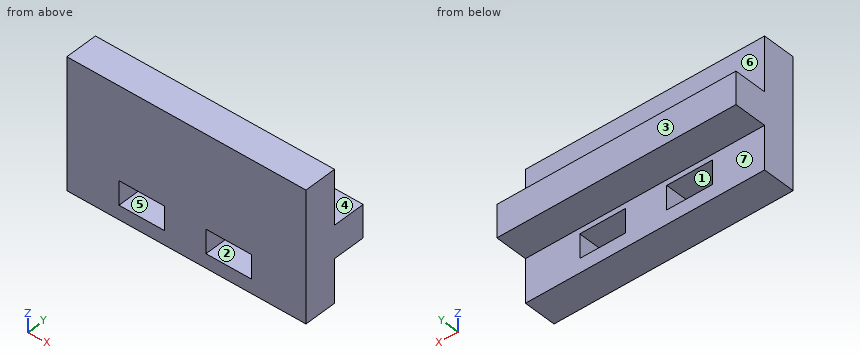
```python
from build123d import *

# Parameters (mm, degrees)
SKETCH_232_W          = 210
SKETCH_232_H          = 53
EXTRUDE_1_DEPTH       = 50
SKETCH_3_W            = 200
SKETCH_3_H            = 43
CUT_EXTRUDE_1_DEPTH   = 45
SKETCH_4_R            = 3.5
EXTRUDE_2_DEPTH       = 2
EXTRUDE_2_TAPER       = 1
FILLET_2_R            = 0.5
SKETCH_4_5_R          = 3.5
EXTRUDE_3_DEPTH       = 2
SKETCH_4_6_R          = 3.5
EXTRUDE_4_DEPTH       = 2
SKETCH_4_7_R          = 3.5
EXTRUDE_5_DEPTH       = 2
FILLET_3_R            = 0.5
FILLET_4_R            = 0.5
FILLET_5_R            = 0.5
SKETCH_7_R            = 6
CUT_EXTRUDE_2_DEPTH   = 14
CUT_EXTRUDE_2_DRAFT   = -5
FILLET_6_R            = 2
SKETCH_8_R            = 7
EXTRUDE_6_DEPTH       = 7
EXTRUDE_6_TAPER       = 5
SKETCH_9_R            = 5.15
CUT_EXTRUDE_3_DEPTH   = 7
CUT_EXTRUDE_3_DRAFT   = 5
SKETCH_10_W           = 29.4
SKETCH_10_H           = 26.3
CUT_EXTRUDE_4_DEPTH   = 5
SKETCH_13_W           = 39.2
SKETCH_13_H           = 27.5
CUT_EXTRUDE_5_DEPTH   = 2
SKETCH_14_W           = 6
SKETCH_14_H           = 6
CUT_EXTRUDE_6_DEPTH   = 5
FILLET_7_R            = 2
EXTRUDE_8_DEPTH       = 3
SKETCH_18_W           = 200
SKETCH_18_H           = 43
SKETCH_18_W_2         = 194
SKETCH_18_H_2         = 37
EXTRUDE_4672_DEPTH    = 3
SKETCH_21_W           = 4.2
SKETCH_21_H           = 2.2
CUT_EXTRUDE_7_DEPTH   = 3
SKETCH_23_OUTSIDE_W   = 255.334
SKETCH_23_OUTSIDE_H   = 98.334
SKETCH_23_OUTSIDE_W_2 = 22
SKETCH_23_OUTSIDE_H_2 = 12
CUT_EXTRUDE_8_DEPTH   = 6


with BuildPart() as part:
    # Sketch 232 → Бобышка-Вытянуть1 (new body)
    with BuildSketch(Plane(origin=(0, 0, 0), x_dir=(1, 0, 0), z_dir=(0, 1, 0))):
        Rectangle(SKETCH_232_W, SKETCH_232_H)
    extrude(amount=EXTRUDE_1_DEPTH)

    # Эскиз3 → Вырез-Вытянуть1 (cut)
    with BuildSketch(Plane.XZ):
        Rectangle(SKETCH_3_W, SKETCH_3_H)
    extrude(amount=-CUT_EXTRUDE_1_DEPTH, mode=Mode.SUBTRACT)

    # Эскиз4 → Бобышка-Вытянуть2 (add)
    with BuildSketch(Plane(origin=(0, 50, 0), x_dir=(1, 0, 0), z_dir=(0, 1, 0))):
        with Locations((98, 19.5)):
            Circle(SKETCH_4_R)
    extrude(amount=EXTRUDE_2_DEPTH, taper=EXTRUDE_2_TAPER)

    # Скругление2
    fillet_2_edges = [part.edges().sort_by_distance(p)[0] for p in [
        (94.53491013, 52, -19.5),
    ]]
    fillet(fillet_2_edges, radius=FILLET_2_R)

    # Эскиз4<5> → Бобышка-Вытянуть3 (add)
    with BuildSketch(Plane(origin=(0, 50, 0), x_dir=(1, 0, 0), z_dir=(0, 1, 0))):
        with Locations(Location((98, -19.5, 0), (0, 0, 90))):
            Circle(SKETCH_4_5_R)
    extrude(amount=EXTRUDE_3_DEPTH)

    # Эскиз4<6> → Бобышка-Вытянуть4 (add)
    with BuildSketch(Plane(origin=(0, 50, 0), x_dir=(1, 0, 0), z_dir=(0, 1, 0))):
        with Locations(Location((-98, -19.5, 0), (0, 0, 270))):
            Circle(SKETCH_4_6_R)
    extrude(amount=EXTRUDE_4_DEPTH)

    # Эскиз4<7> → Бобышка-Вытянуть5 (add)
    with BuildSketch(Plane(origin=(0, 50, 0), x_dir=(1, 0, 0), z_dir=(0, 1, 0))):
        with Locations(Location((-98, 19.5, 0), (0, 0, 90))):
            Circle(SKETCH_4_7_R)
    extrude(amount=EXTRUDE_5_DEPTH)

    # Скругление3
    fillet_3_edges = [part.edges().sort_by_distance(p)[0] for p in [
        (-98, 52, 16),
    ]]
    fillet(fillet_3_edges, radius=FILLET_3_R)

    # Скругление4
    fillet_4_edges = [part.edges().sort_by_distance(p)[0] for p in [
        (-98, 52, -16),
    ]]
    fillet(fillet_4_edges, radius=FILLET_4_R)

    # Скругление5
    fillet_5_edges = [part.edges().sort_by_distance(p)[0] for p in [
        (98, 52, 23),
    ]]
    fillet(fillet_5_edges, radius=FILLET_5_R)


with BuildPart() as cut_extrude_2_tool:
    # Эскиз7 → Вырез-Вытянуть2 (with draft: the straight prism first)
    with BuildSketch(Plane(origin=(0, 0, -26.5), x_dir=(-1, 0, 0), z_dir=(0, 0, -1))):
        with Locations((0, 35.081888724)):
            Circle(SKETCH_7_R)
    extrude(amount=-CUT_EXTRUDE_2_DEPTH)
    # Вырез-Вытянуть2: the draft: its side faces are tilted about the plane it starts from
    cut_extrude_2_sides = [cut_extrude_2_tool.faces().sort_by_distance(p)[0] for p in [
        (6, 35.081888724, -19.5),
    ]]
    draft(cut_extrude_2_sides, Plane(origin=(0, 0, -26.5), x_dir=(-1, 0, 0), z_dir=(0, 0, -1)), CUT_EXTRUDE_2_DRAFT)


with BuildPart() as part_1:
    add(part.part)

    # Вырез-Вытянуть2: cut by cut_extrude_2_tool
    add(cut_extrude_2_tool.part, mode=Mode.SUBTRACT)

    # Скругление6
    fillet_6_edges = [part_1.edges().sort_by_distance(p)[0] for p in [
        (6, 35.081888724, -26.5),
    ]]
    fillet(fillet_6_edges, radius=FILLET_6_R)

    # Эскиз8 → Бобышка-Вытянуть6 (add)
    with BuildSketch(Plane.XY.offset(-21.5)):
        with Locations((0, 35.081888724)):
            Circle(SKETCH_8_R)
    extrude(amount=EXTRUDE_6_DEPTH, taper=EXTRUDE_6_TAPER)


with BuildPart() as cut_extrude_3_tool:
    # Эскиз9 → Вырез-Вытянуть3 (with draft: the straight prism first)
    with BuildSketch(Plane.XY.offset(-14.5)):
        with Locations((0, 35.081888724)):
            Circle(SKETCH_9_R)
    extrude(amount=-CUT_EXTRUDE_3_DEPTH)
    # Вырез-Вытянуть3: the draft: its side faces are tilted about the plane it starts from
    cut_extrude_3_sides = [cut_extrude_3_tool.faces().sort_by_distance(p)[0] for p in [
        (-5.15, 35.081888724, -18),
    ]]
    draft(cut_extrude_3_sides, Plane.XY.offset(-14.5), CUT_EXTRUDE_3_DRAFT)


with BuildPart() as part_2:
    add(part_1.part)

    # Вырез-Вытянуть3: cut by cut_extrude_3_tool
    add(cut_extrude_3_tool.part, mode=Mode.SUBTRACT)

    # Эскиз10 → Вырез-Вытянуть4 (cut)
    with BuildSketch(Plane.XY.offset(26.5)):
        with Locations((-50, 25)):
            Rectangle(SKETCH_10_W, SKETCH_10_H)
    extrude(amount=-CUT_EXTRUDE_4_DEPTH, mode=Mode.SUBTRACT)

    # Эскиз13 → Вырез-Вытянуть5 (cut)
    with BuildSketch(Plane(origin=(0, 0, 21.5), x_dir=(-1, 0, 0), z_dir=(0, 0, -1))):
        with Locations((50, 25)):
            Rectangle(SKETCH_13_W, SKETCH_13_H)
    extrude(amount=-CUT_EXTRUDE_5_DEPTH, mode=Mode.SUBTRACT)

    # Эскиз14 → Вырез-Вытянуть6 (cut)
    with BuildSketch(Plane.XY.offset(26.5)):
        with Locations((-76.5, 31.8)):
            Rectangle(SKETCH_14_W, SKETCH_14_H)
        with Locations((-76.5, 18.2)):
            Rectangle(SKETCH_14_W, SKETCH_14_H)
    extrude(amount=-CUT_EXTRUDE_6_DEPTH, mode=Mode.SUBTRACT)

    # Скругление7
    fillet_7_edges = [part_2.edges().sort_by_distance(p)[0] for p in [
        (-105, 50, 0),
        (0, 50, 26.5),
        (105, 50, 0),
        (105, 25, 26.5),
        (-105, 25, 26.5),
        (-105, 25, -26.5),
        (105, 25, -26.5),
        (0, 50, -26.5),
    ]]
    fillet(fillet_7_edges, radius=FILLET_7_R)


with BuildPart() as body_2:
    # Эскиз17 → Бобышка-Вытянуть8 (new body)
    with BuildSketch(Plane.XZ):
        with BuildLine():
            Line((-105, 24.5), (-105, -24.5))
            ThreePointArc((-105, -24.5), (-104.414213562, -25.914213562), (-103, -26.5))
            Line((-103, -26.5), (103, -26.5))
            ThreePointArc((103, -26.5), (104.414213562, -25.914213562), (105, -24.5))
            Line((105, -24.5), (105, 24.5))
            ThreePointArc((105, 24.5), (104.414213562, 25.914213562), (103, 26.5))
            Line((103, 26.5), (-103, 26.5))
            ThreePointArc((-103, 26.5), (-104.414213562, 25.914213562), (-105, 24.5))
        make_face()
    extrude(amount=EXTRUDE_8_DEPTH)

    # Эскиз18 → Extrude 4672 (add)
    with BuildSketch(Plane(origin=(0, 0, 0), x_dir=(1, 0, 0), z_dir=(0, 1, 0))):
        Rectangle(SKETCH_18_W, SKETCH_18_H)
        Rectangle(SKETCH_18_W_2, SKETCH_18_H_2, mode=Mode.SUBTRACT)
    extrude(amount=EXTRUDE_4672_DEPTH)

    # Эскиз21 → Вырез-Вытянуть7 (cut)
    with BuildSketch(Plane.XZ.offset(3)):
        with Locations((10.5, 16.9)):
            Rectangle(SKETCH_21_W, SKETCH_21_H)
        with Locations((18.5, 16.9)):
            Rectangle(SKETCH_21_W, SKETCH_21_H)
    extrude(amount=-CUT_EXTRUDE_7_DEPTH, mode=Mode.SUBTRACT)

    # Эскиз23 outside → Вырез-Вытянуть8 (cut)
    with BuildSketch(Plane.XZ.offset(3)):
        Rectangle(SKETCH_23_OUTSIDE_W, SKETCH_23_OUTSIDE_H)
        with Locations((14.6, 20.5)):
            Rectangle(SKETCH_23_OUTSIDE_W_2, SKETCH_23_OUTSIDE_H_2, mode=Mode.SUBTRACT)
    extrude(amount=-CUT_EXTRUDE_8_DEPTH, mode=Mode.SUBTRACT)


solid = body_2.part
```
Check sheet for the modelled part. Datum: model origin and axes. Units: mm. Face numbers are marked on the shaded views. A direction names the side the tool comes from. Round coordinates to 2 decimals unless told otherwise and drop trailing zeros. Write each loop counter-clockwise with the first axis right and the second up, starting at its lowest first coordinate (ties: lowest second). Pieces come first, ordered by that corner, then holes. Notation, with made-up numbers: M 80.25,-1.5 L 118.25,-1.5 A26 cw 118.25,29.5 Z; hole C -10,9 d11. An arc over 180 degrees is marked long. Write item = value, one per line. Start each with the question number.
1. Gauge pin test, flat ends, axial feed: pin 1 (1.5 mm diameter, centred on x = 16, y = 1, fed in from -Z); pin 2 (1.5 mm diameter, centred on x = 20, z = 24, fed in from +Y). Record the tip position at first contact, or that the pin passes through.
2. Section check D-D, the plane x = 6.25. Record the cut outline in (y, z), then the cut area to 3 significant figures.
3. Section check C-C, the plane z = 16.5. Record the cut outline in (x, y).
4. Release check for a two-part mould opening along Z. For the marked faces 1, 2, 3 and 4 record: pulls with the +Z half, pulls with the -Z half, needs draft (parallel to the pull), parting line crosses it, or undercut.
5. Tool access check on the marked faces 5, 6 and 7. Record the directions out of +Z, -Z, +X, -X, +Y, -Y that give a thin tool (end or side, any length) a straight path to the whole face; none if there is none.
6. Scan lines: line 1 (Z direction, x = 17.25, y = -0.15); line 2 (X direction, y = -0.2, z = 16.5); line 3 (Z direction, x = 6.75, y = 0.7). Record each from-to range of solid material in increasing order. Write a range as [from, to].
7. Section check B-B, the plane x = 10.5. Record the cut outline in (y, z).
8. Section check A-A, the plane y = -0.8. Record the cut outline in (x, z), then the cut area to 3 significant figures.
Results found:
q1.pin_1 = 18.5
q1.pin_2 = 0
q2.outline = M -3,14.5 L 0,14.5 L 0,18.5 L 3,18.5 L 3,21.5 L 0,21.5 L 0,26.5 L -3,26.5 Z
q2.area = 45.0 mm^2
q3.outline = M 3.6,-3 L 8.4,-3 L 8.4,0 L 3.6,0 Z; M 12.6,-3 L 16.4,-3 L 16.4,0 L 12.6,0 Z; M 20.6,-3 L 25.6,-3 L 25.6,0 L 20.6,0 Z
q4.face_1 = undercut
q4.face_2 = undercut
q4.face_3 = needs draft
q4.face_4 = pulls with the +Z half
q5.face_5 = +Y, -Y
q5.face_6 = +Z, +X, -X, +Y
q5.face_7 = -Z, +X, -X, +Y
q6.line_1 = [14.5, 15.8], [18, 26.5]
q6.line_2 = [3.6, 8.4], [12.6, 16.4], [20.6, 25.6]
q6.line_3 = [18.5, 21.5]
q7.outline = M -3,14.5 L 0,14.5 L 0,15.8 L -3,15.8 Z; M -3,18 L 0,18 L 0,18.5 L 3,18.5 L 3,21.5 L 0,21.5 L 0,26.5 L -3,26.5 Z
q8.outline = M 3.6,14.5 L 25.6,14.5 L 25.6,26.5 L 3.6,26.5 Z; hole M 8.4,15.8 L 12.6,15.8 L 12.6,18 L 8.4,18 Z; hole M 16.4,15.8 L 20.6,15.8 L 20.6,18 L 16.4,18 Z
q8.area = 246 mm^2
